The model under review builds one solid part; all positions refer to its coordinate system, in mm. A direction names the side the tool comes from. Coordinates: 2 decimals unless noted, no trailing zeros. Write each loop counter-clockwise with the first axis right and the second up, starting at its lowest first coordinate (ties: lowest second). Pieces come first, ordered by that corner, then holes.
1) Machinability: for faces 4 (the flat face through (0.089, -43.043, 106.834)), 5 (the cylindrical face through (0.09, -0.66, 235.45)), which of the approach directions +Z, -Z, +X, -X, +Y, -Y give a long, thin tool a straight path to every point of the face, cutting with its end or side? Answer none if there is none.
2) For P1, Ø2, axis at x = 2.5, z = 103, coming from the +Y side; P2, Ø4, axis at x = 0, y = 21, coming from the +Z side; P3, Ø1.5, axis at x = -2, z = 101.5, coming from the -Y side, all flat-tipped, find the tip position at first contact; note any pin that passes through.
3) Add section A-A, the plane y = 0. State the section outline as (x, z) points, then the cut area to 3 significant figures.
4) Add section C-C, the plane x = -4.25. State the section outline as (y, z) points (3 decimals).
5) Add section B-B, the plane z = 0. State the section outline as (x, y) points, then the cut area to 3 significant figures.
6) Mouldability with a two-part tool opening along Z and no side actions: class faces 1 (the flat face through (0.09, 39.88, 106.57)), 2 (the flat face through (6.35, 42, 94)), 3 (the cylindrical face through (0.089, 0.728, 238.625)) as released by +Z, released by -Z, zero draft, split by the parting line, or undercut.
7) For line 1 (Y direction, x = 3.5, z = 0); line 2 (Z direction, x = 2.5, y = 0); line 3 (Y direction, x = -3.5, z = 181), list the stretches that pass through material, from the lowest coordinate up.
from build123d import *

# Parameters (mm, degrees)
F1_DEPTH = 6.35


with BuildPart() as f1:
    # F0 (on Right) → F1 (new body, symmetric)
    with BuildSketch(Plane.YZ):
        with BuildLine():
            Line((-34.806537, 206.582127), (-51.513675, 4.253708))
            ThreePointArc((-51.513675, 4.253708), (0, -51.689), (51.513675, 4.253708))
            Line((51.513675, 4.253708), (34.806537, 206.582127))
            ThreePointArc((34.806537, 206.582127), (0, 238.633), (-34.806537, 206.582127))
        make_face()
        with BuildLine():
            ThreePointArc((48.349444, 3.992424), (0, -48.514), (-48.349444, 3.992424))
            Line((-48.349444, 3.992424), (-31.642306, 206.320843))
            ThreePointArc((-31.642306, 206.320843), (0, 235.458), (31.642306, 206.320843))
            Line((31.642306, 206.320843), (48.349444, 3.992424))
        make_face(mode=Mode.SUBTRACT)
    extrude(amount=F1_DEPTH, both=True)


solid = f1.part
Geometry results:
1. face 4: +Z, +X, -X, -Y
1. face 5: +X, -X
2. P1: stops at y = 43.44
2. P2: stops at z = 233.01
2. P3: stops at y = -43.55
3. outline: (-6.35, -51.69) - (6.35, -51.69) - (6.35, -48.51) - (-6.35, -48.51) - close; (-6.35, 235.46) - (6.35, 235.46) - (6.35, 238.63) - (-6.35, 238.63) - close
3. area: 80.6 mm2
4. outline: (-51.514, 4.254) arc R51.689 ccw (long way) to (51.514, 4.254) - (34.807, 206.582) arc R34.925 ccw to (-34.807, 206.582) - close; hole (-48.349, 3.992) arc R48.514 ccw (long way) to (48.349, 3.992) - (31.642, 206.321) arc R31.75 ccw to (-31.642, 206.321) - close
5. outline: (-6.35, -51.69) - (6.35, -51.69) - (6.35, -48.51) - (-6.35, -48.51) - close; (-6.35, 48.51) - (6.35, 48.51) - (6.35, 51.69) - (-6.35, 51.69) - close
5. area: 80.6 mm2
6. face 1: undercut
6. face 2: zero draft
6. face 3: released by +Z
7. line 1: y = -51.69 to -48.51, 48.51 to 51.69
7. line 2: z = -51.69 to -48.51, 235.46 to 238.63
7. line 3: y = -36.92 to -33.73, 33.73 to 36.92
